Verification items for the finished model (mm, model axes). A direction names the side the tool comes from. Give positions to 0.01 mm unless a question says otherwise; leave off trailing zeros. Loops run counter-clockwise (first coordinate to the right, second up) from the corner with the lowest first, then second, coordinate; pieces in that order, holes last. Notation, with made-up numbers: (29.5, 82) - (56.5, 82) arc R22 cw to (56.5, 89) - close; hole circle Ø8 at (83, 36). An arc over 180 degrees is marked (long way). One line per question, with ' | ' between items. Start each with the question number.
1. Section check C-C, the plane y = -4. Enter the section's corners in (x, z), then the cut area to 3 significant figures.
2. Depth check by flat-ended pin: pin 1 Ø2 at (x, y) = (0, 1.5) entering from -Z. Enter the tip coordinate at first touch or a pass-through.
3. Tool access check on faces 5 (the face through (-2.371, 0, 5)), 6 (the face through (4.629, 0, 11)). Record the directions out of +Z, -Z, +X, -X, +Y, -Y that give a thin tool (end or side, any length) a straight path to the whole face; none if there is none.
4. Mould release check, pull along Y, two halves, no side actions. Record for faces 1 (the face through (1, 0, 10)), 2 (the face through (0, 7.499, 6)), 3 (the face through (1, 4.499, 5)), 4 (the face through (-5.371, 0, 6)): +Y half, -Y half, draft (parallel to the pull), parting line (faces both ways), or undercut.
5. Section check B-B, the plane x = -1.75. Enter the section's corners in (y, z), then the cut area to 3 significant figures.
6. Section check A-A, the plane z = 7.5. Enter the section's corners in (x, y), then the cut area to 3 significant figures.
7. Thickness scan on line 1 along Y through (x, z) = (-0.75, 3); line 2 along Z through (x, y) = (0.75, 0); line 3 along X through (y, z) = (2.25, 8.5). Record the ranges inside material, lowest first. Write a range as from..to.
Autodesk Inventor part; units mm, degrees
ref_plane "YZ Plane" through (0, 0, 0) normal (1, 0, 0) x (0, 1, 0)
ref_plane "XZ Plane" through (0, 0, 0) normal (0, 1, 0) x (-1, 0, 0)
ref_plane "XY Plane" through (0, 0, 0) normal (0, 0, 1) x (1, 0, 0)
sketch "Эскиз1" plane through (0, 0, 0) normal (0, 0, 1) x (1, 0, 0)
  line L0 (4.6286, 7.4989) -> (-5.3714, 7.4989)
  line L1 (-5.3714, 7.4989) -> (-5.3714, -7.7011)
  line L2 (-5.3714, -7.7011) -> (4.6286, -7.7011)
  line L3 (4.6286, -7.7011) -> (4.6286, -4.7011)
  line L4 (4.6286, -4.7011) -> (-2.3714, -4.7011)
  line L5 (-2.3714, 4.4989) -> (4.6286, 4.4989)
  line L6 (4.6286, 4.4989) -> (4.6286, 7.4989)
  line L7 (-2.3714, 4.4989) -> (-2.3714, -4.7011)
  point P0 (0, 0)
  dimension "d1" = 9.2
  dimension "d2" = 3
  dimension "d3" = 3
  dimension "d4" = 3
  dimension "d7" = 10
extrude "Выдавливание1" add sketch "Эскиз1" along normal blind 10
sketch "Эскиз3" plane through (0, 0, 10) normal (0, 0, 1) x (1, 0, 0)
  line L0 (4.6286, 7.4989) -> (-5.3714, 7.4989)
  line L1 (4.6286, -7.7011) -> (4.6286, -4.7011)
  line L2 (-5.3714, 7.4989) -> (4.6286, 7.4989)
  line L3 (4.6286, 7.4989) -> (4.6286, -7.7011)
  line L4 (4.6286, -7.7011) -> (-5.3714, -7.7011)
  line L5 (-5.3714, -7.7011) -> (-5.3714, 7.4989)
  point P0 (0, 0)
  point P1 (4.6286, 7.4989)
extrude "Выдавливание3" add sketch "Эскиз3" along normal blind 2
properties part number "ограничитель"
Results list:
1) outline: (-5.37, 0) - (-2.37, 0) - (-2.37, 10) - (4.63, 10) - (4.63, 12) - (-5.37, 12) - close | area: 50.0 mm²
2) pin 1: z = 10
3) face 5: -Z, +X | face 6: +Z, -Z, +X, +Y, -Y
4) face 1: undercut | face 2: +Y half | face 3: undercut | face 4: draft
5) outline: (-7.7, 0) - (-4.7, 0) - (-4.7, 10) - (4.5, 10) - (4.5, 0) - (7.5, 0) - (7.5, 12) - (-7.7, 12) - close | area: 90.4 mm²
6) outline: (-5.37, -7.7) - (4.63, -7.7) - (4.63, -4.7) - (-2.37, -4.7) - (-2.37, 4.5) - (4.63, 4.5) - (4.63, 7.5) - (-5.37, 7.5) - close | area: 87.6 mm²
7) line 1: -7.7..-4.7, 4.5..7.5 | line 2: 10..12 | line 3: -5.37..-2.37
